CAD build for the part. Positions are in the model's coordinates, mm. Face numbers are marked on the shaded views. A direction names the side the tool comes from. Round coordinates to 2 decimals unless told otherwise and drop trailing zeros. Order: outer loops, then holes, each group sorted by start corner. A loop starts at its lowest first (then second) coordinate and runs counter-clockwise, first axis right, second up. Notation, with made-up numbers: (0.25, 81.5) -> (53.25, 81.5) arc R29 ccw to (53.25, 113.5) -> close; hole circle Ø4 at (45.25, 62.25). An arc over 180 degrees is marked (long way). Return JSON: item names as keys, results as strings. Group by question number.
Q1. Cut at C-C (z = 100.5). Write the cut outline in (x, y), then the cut area to 3 significant figures.
Q2. Cut at B-B (x = 5.25). Write the cut outline in (y, z).
Q3. Probe line 1 along Y through (x, z) = (2.75, 3.5); line 2 along Z through (x, y) = (7.5, -1); line 3 along Z through (x, y) = (4, -15). List the from-to ranges inside material, lowest first.
Q4. Which spindle directions (+Z, -Z, +X, -X, +Y, -Y) get a long thin tool onto all of the face, cutting with end or side? Do the marked faces 4 and 5. Say none if no direction does.
Q5. Flat gauge pin, fed straight in: pin 1 (3 mm diameter, centred on x = 1, y = 13.5, fed in from +Z). Where does the tip first touch, or does it go through?
Q6. Mould opens along Z. For the marked faces 1, 2 and 3 say: +Z half, -Z half, draft (parallel to the pull), parting line (faces both ways), or undercut.
Q7. Cut at A-A (y = 0). Write the cut outline in (x, z).
Autodesk Inventor part; units mm, degrees
ref_plane "YZ Plane" through (0, 0, 0) normal (1, 0, 0) x (0, 1, 0)
ref_plane "XZ Plane" through (0, 0, 0) normal (0, 1, 0) x (-1, 0, 0)
ref_plane "XY Plane" through (0, 0, 0) normal (0, 0, 1) x (1, 0, 0)
sketch "Sketch1" plane through (0, 0, 0) normal (1, 0, 0) x (0, 1, 0)
  arc A0 (-19.1008, 0) -> (19.1008, 0) centre (0, 0) ccw
  arc A1 (19.1008, 115.5112) -> (-19.1008, 115.5112) centre (0, 115.5112) ccw
  line L0 (19.1008, 115.5112) -> (19.1008, 0)
  line L1 (-19.1008, 0) -> (-19.1008, 115.5112)
  arc A2 (-17.5133, 0) -> (17.5133, 0) centre (0, 0) ccw
  line L2 (-17.5133, 0) -> (-17.5133, 115.5112)
  arc A3 (17.5133, 115.5112) -> (-17.5133, 115.5112) centre (0, 115.5112) ccw
  line L3 (17.5133, 115.5112) -> (17.5133, 0)
  dimension "d0" = 19.1008
  dimension "d1" = 115.5112
  dimension "d5" = 1.5875
extrude "Extrusion1" add sketch "Sketch1" along normal blind 9
properties part number "STANDIN,BELT,70T,HTD5mm" material "Nylon 6/6"
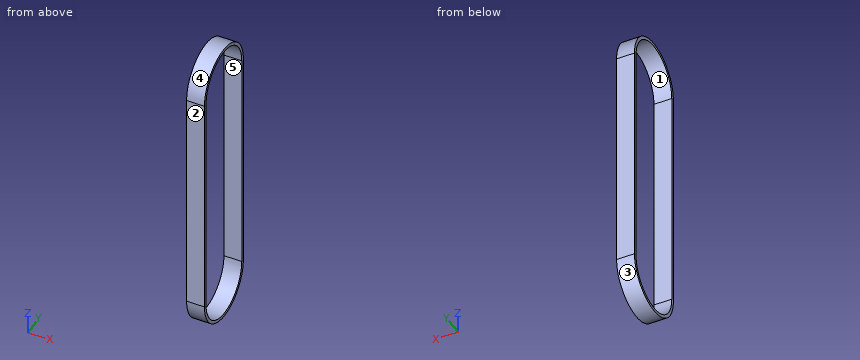
Solution:
{
 "1": {"outline": "(0, -19.1) -> (9, -19.1) -> (9, -17.51) -> (0, -17.51) -> close; (0, 17.51) -> (9, 17.51) -> (9, 19.1) -> (0, 19.1) -> close", "area": "28.6 mm²"},
 "2": {"outline": "(-19.1, 0) arc R19.1 ccw to (19.1, 0) -> (19.1, 115.51) arc R19.1 ccw to (-19.1, 115.51) -> close; hole (-17.51, 0) arc R17.51 ccw to (17.51, 0) -> (17.51, 115.51) arc R17.51 ccw to (-17.51, 115.51) -> close"},
 "3": {"line 1": "y = -19.1 to -17.51, 17.51 to 19.1", "line 2": "z = -19.07 to -17.48, 133 to 134.59", "line 3": "z = -11.83 to -9.04, 124.55 to 127.34"},
 "4": {"face 4": "+Z, +X, -X", "face 5": "+X, -X"},
 "5": {"pin 1": "stops at z = 130.37"},
 "6": {"face 1": "undercut", "face 2": "draft", "face 3": "-Z half"},
 "7": {"outline": "(0, -19.1) -> (9, -19.1) -> (9, -17.51) -> (0, -17.51) -> close; (0, 133.02) -> (9, 133.02) -> (9, 134.61) -> (0, 134.61) -> close"}
}
